Work out the finished part from the listing and answer in its coordinate system (mm). Face numbers are marked on the shaded views. A direction names the side the tool comes from. Round coordinates to 2 decimals unless told otherwise and drop trailing zeros. Loops run counter-clockwise (first coordinate to the right, second up) from the corner with the lowest first, then second, coordinate; pieces in that order, holes last.
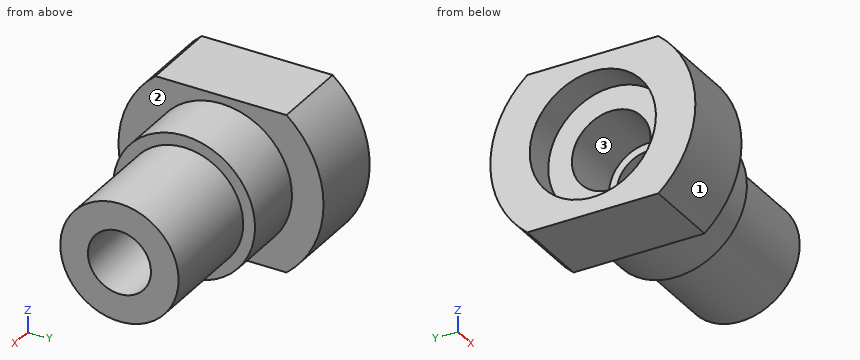
```python
from build123d import *

# Parameters (mm, degrees)
CUT_EXTRUDE_1_DEPTH = 15.335271187


with BuildPart() as part:
    # Эскиз1 → Повернуть1 (revolve)
    with BuildSketch(Plane.XY, mode=Mode.PRIVATE) as revolve_1_sk:
        Polygon((0, 4), (2, 4), (2, 2.5), (6, 2.5), (6, 2), (16, 2), (16, 3.75), (9, 3.75), (9, 4.5), (5, 4.5), (5, 6.5), (0, 6.5), align=None)
    revolve(revolve_1_sk.sketch.rotate(Axis((0, 0, 0), (1, 0, 0)), 90), axis=Axis((0, 0, 0), (1, 0, 0)))

    # Эскиз2 → Вырез-Вытянуть1 (cut, through all)
    with BuildSketch(Plane(origin=(5, 0, 0), x_dir=(0, 0, -1), z_dir=(1, 0, 0))):
        with BuildLine():
            ThreePointArc((-5, 4.153311931), (-6.5, 0), (-5, -4.153311931))
            Line((-5, -4.153311931), (-5, 4.153311931))
        make_face()
        with BuildLine():
            Line((5, 4.153311931), (5, -4.153311931))
            ThreePointArc((5, -4.153311931), (6.11350963, -2.207940217), (6.5, 0))
            ThreePointArc((6.5, 0), (6.11350963, 2.207940217), (5, 4.153311931))
        make_face()
    extrude(amount=-CUT_EXTRUDE_1_DEPTH, mode=Mode.SUBTRACT)


solid = part.part
```
1. Given pin 1 (3 mm diameter, centred on x = 7.5, z = 0.5, fed in from -Y); pin 2 (5 mm diameter, centred on x = 4, z = 4, fed in from -Y); pin 3 (2.5 mm diameter, centred on y = 1, z = 0, fed in from -X); pin 4 (3.5 mm diameter, centred on y = 0, z = 0, fed in from +X), each flat-ended and moving along its own axis, determine where each tip first touches the part or whether it passes through.
Answer key:
pin 1: stops at y = -4.5
pin 2: stops at y = -6.32
pin 3: stops at x = 6
pin 4: passes through
2. Find section D-D (z = 3.25). Write down the section's boundary in (x, y), then the cut area to 3 significant figures.
Answer key:
outline: (0, -5.63) - (5, -5.63) - (5, -3.11) - (9, -3.11) - (9, -1.87) - (16, -1.87) - (16, 1.87) - (9, 1.87) - (9, 3.11) - (5, 3.11) - (5, 5.63) - (0, 5.63) - (0, 2.33) - (2, 2.33) - (2, -2.33) - (0, -2.33) - close
area: 98.1 mm2
3. Find section B-B (z = 0). Write down the section's boundary in (x, y).
Answer key:
outline: (0, -6.5) - (5, -6.5) - (5, -4.5) - (9, -4.5) - (9, -3.75) - (16, -3.75) - (16, -2) - (6, -2) - (6, -2.5) - (2, -2.5) - (2, -4) - (0, -4) - close; (0, 4) - (2, 4) - (2, 2.5) - (6, 2.5) - (6, 2) - (16, 2) - (16, 3.75) - (9, 3.75) - (9, 4.5) - (5, 4.5) - (5, 6.5) - (0, 6.5) - close
4. Consider probe 1 along Y at (x, z) = (1.2, 0); probe 2 along Y at (x, z) = (4.5, 0); probe 3 along X at (y, z) = (2.75, 3). Determine where each line is inside the solid, lowest interval first.
Answer key:
probe 1: y = -6.5 to -4, 4 to 6.5
probe 2: y = -6.5 to -2.5, 2.5 to 6.5
probe 3: x = 0 to 9
5. Which of the six approach directions +Z, -Z, +X, -X, +Y, -Y give full straight-line access (tool end or side, diameter ignored) to the marked faces 1, 2 and 3?
Answer key:
face 1: +X, -X, -Y
face 2: +X
face 3: -X
6. Find section A-A (y = 0). Write down the section's boundary in (x, z).
Answer key:
outline: (0, -5) - (5, -5) - (5, -4.5) - (9, -4.5) - (9, -3.75) - (16, -3.75) - (16, -2) - (6, -2) - (6, -2.5) - (2, -2.5) - (2, -4) - (0, -4) - close; (0, 4) - (2, 4) - (2, 2.5) - (6, 2.5) - (6, 2) - (16, 2) - (16, 3.75) - (9, 3.75) - (9, 4.5) - (5, 4.5) - (5, 5) - (0, 5) - close
7. Find section C-C (x = 3.5). Write down the section's boundary in (y, z), then the cut area to 3 significant figures.
Answer key:
outline: (-4.15, -5) - (4.15, -5) arc R6.5 ccw to (4.15, 5) - (-4.15, 5) arc R6.5 ccw to start; hole circle Ø5 at (0, 0)
area: 96.1 mm2
